```python
from build123d import *

# Parameters (mm, degrees)
F1_DEPTH = 3.048


with BuildPart() as f1:
    # F0 (on Front) → F1 (new body)
    with BuildSketch(Plane.XZ):
        with BuildLine():
            Line((-9.525, 114.3), (-15.7474569047, 65.5082893304))
            ThreePointArc((-15.7474569047, 65.5082893304), (-10.4912828548, 75.4142187767), (0, 79.375))
            Line((0, 79.375), (0, 104.775))
            ThreePointArc((0, 104.775), (-6.7351920908, 107.5648079092), (-9.525, 114.3))
        make_face()
        with BuildLine():
            Line((0, 104.775), (0, 79.375))
            ThreePointArc((0, 79.375), (10.4912828548, 75.4142187767), (15.7474569047, 65.5082893304))
            Line((15.7474569047, 65.5082893304), (9.525, 114.3))
            ThreePointArc((9.525, 114.3), (6.7351920908, 107.5648079092), (0, 104.775))
        make_face()
        with BuildLine():
            ThreePointArc((9.525, 114.3), (0, 123.825), (-9.525, 114.3))
            ThreePointArc((-9.525, 114.3), (-6.7351920908, 107.5648079092), (0, 104.775))
            ThreePointArc((0, 104.775), (6.7351920908, 107.5648079092), (9.525, 114.3))
        make_face()
        with BuildLine():
            ThreePointArc((3.175, 114.3), (2.2450640303, 112.0549359697), (0, 111.125))
            ThreePointArc((0, 111.125), (-2.2450640303, 116.5450640303), (3.175, 114.3))
        make_face(mode=Mode.SUBTRACT)
        with BuildLine():
            ThreePointArc((-15.7474569047, 61.4917106696), (-10.4912828548, 51.5857812233), (0, 47.625))
            Line((0, 47.625), (0, 60.325))
            ThreePointArc((0, 60.325), (-3.175, 63.5), (0, 66.675))
            Line((0, 66.675), (0, 79.375))
            ThreePointArc((0, 79.375), (-10.4912828548, 75.4142187767), (-15.7474569047, 65.5082893304))
            ThreePointArc((-15.7474569047, 65.5082893304), (-15.875, 63.5), (-15.7474569047, 61.4917106696))
        make_face()
        with BuildLine():
            ThreePointArc((-9.525, 0), (-6.7351920908, 6.7351920908), (0, 9.525))
            Line((0, 9.525), (0, 47.625))
            ThreePointArc((0, 47.625), (-10.4912828548, 51.5857812233), (-15.7474569047, 61.4917106696))
            Line((-15.7474569047, 61.4917106696), (-9.525, 0))
        make_face()
        with BuildLine():
            Line((0, 47.625), (0, 9.525))
            ThreePointArc((0, 9.525), (6.7351920908, 6.7351920908), (9.525, 0))
            Line((9.525, 0), (36.5125, 0))
            ThreePointArc((36.5125, 0), (38.8373399243, 5.6126600757), (44.45, 7.9375))
            Line((44.45, 7.9375), (17.9461215627, 7.9375))
            ThreePointArc((17.9461215627, 7.9375), (11.9794807993, 10.6336655463), (10.0597951449, 16.8934512966))
            Line((10.0597951449, 16.8934512966), (15.7474569047, 61.4917106696))
            ThreePointArc((15.7474569047, 61.4917106696), (10.4912828548, 51.5857812233), (0, 47.625))
        make_face()
        with BuildLine():
            ThreePointArc((3.175, 0), (-2.2450640303, -2.2450640303), (0, 3.175))
            Line((0, 3.175), (0, 9.525))
            ThreePointArc((0, 9.525), (-6.7351920908, 6.7351920908), (-9.525, 0))
            ThreePointArc((-9.525, 0), (-6.7351920908, -6.7351920908), (0, -9.525))
            Line((0, -9.525), (0.6794904459, -9.5007324841))
            ThreePointArc((0.6794904459, -9.5007324841), (6.9712901065, -6.4905114784), (9.525, 0))
            Line((9.525, 0), (3.175, 0))
        make_face()
        with BuildLine():
            Line((0, 9.525), (0, 3.175))
            ThreePointArc((0, 3.175), (2.2450640303, 2.2450640303), (3.175, 0))
            Line((3.175, 0), (9.525, 0))
            ThreePointArc((9.525, 0), (6.7351920908, 6.7351920908), (0, 9.525))
        make_face()
        with BuildLine():
            Line((36.5125, 0), (9.525, 0))
            ThreePointArc((9.525, 0), (6.9712901065, -6.4905114784), (0.6794904459, -9.5007324841))
            Line((0.6794904459, -9.5007324841), (44.45, -7.9375))
            ThreePointArc((44.45, -7.9375), (38.8373399243, -5.6126600757), (36.5125, 0))
        make_face()
        with BuildLine():
            ThreePointArc((44.45, 7.9375), (38.8373399243, 5.6126600757), (36.5125, 0))
            ThreePointArc((36.5125, 0), (38.8373399243, -5.6126600757), (44.45, -7.9375))
            ThreePointArc((44.45, -7.9375), (50.0626600757, -5.6126600757), (52.3875, 0))
            ThreePointArc((52.3875, 0), (50.0626600757, 5.6126600757), (44.45, 7.9375))
        make_face()
        with BuildLine():
            ThreePointArc((47.625, 0), (44.45, -3.175), (41.275, 0))
            ThreePointArc((41.275, 0), (44.45, 3.175), (47.625, 0))
        make_face(mode=Mode.SUBTRACT)
        with BuildLine():
            Line((0, 60.325), (0, 47.625))
            ThreePointArc((0, 47.625), (10.4912828548, 51.5857812233), (15.7474569047, 61.4917106696))
            ThreePointArc((15.7474569047, 61.4917106696), (15.8430821396, 62.4938323604), (15.875, 63.5))
            ThreePointArc((15.875, 63.5), (15.8430821396, 64.5061676396), (15.7474569047, 65.5082893304))
            ThreePointArc((15.7474569047, 65.5082893304), (10.4912828548, 75.4142187767), (0, 79.375))
            Line((0, 79.375), (0, 66.675))
            ThreePointArc((0, 66.675), (2.2450640303, 65.7450640303), (3.175, 63.5))
            ThreePointArc((3.175, 63.5), (2.2450640303, 61.2549359697), (0, 60.325))
        make_face()
    extrude(amount=F1_DEPTH)


solid = f1.part
```
Check sheet for the modelled part. Datum: model origin and axes. Units: mm. A direction names the side the tool comes from. Give positions to 0.01 mm unless a question says otherwise; leave off trailing zeros. Write each loop counter-clockwise with the first axis right and the second up, starting at its lowest first coordinate (ties: lowest second). Pieces come first, ordered by that corner, then holes. Notation, with made-up numbers: (-18, 30.25) -> (24, 30.25) arc R11 ccw to (24, 36.25) -> close; hole circle Ø3 at (89, 75). An arc over 180 degrees is marked (long way). Use CSV: the item, a comma, the result in double quotes. Start each with the question number.
Q1. Cross-section at C-C on z = 53. Enter the section's corners in (x, y).
Q2. Release check for a two-part mould opening along Z. For faces 1 (the flat face through (3, -3.048, 43)), 2 (the flat face through (12.864, -1.503, 38.88)), 3 (the flat face through (-12.6, -1.5, 90.2)) record: +Z half, -Z half, draft (parallel to the pull), parting line (faces both ways), or undercut.
Q3. Depth check by flat-ended pin: P1, Ø5, axis at x = 0, z = 114.3, coming from the +Y side. Enter the tip coordinate at first touch or a pass-through.
Q4. Cross-section at B-B on x = 38.5. Enter the section's corners in (y, z), and give its area (3 significant figures).
Q5. Tool access check on faces 4 (the flat face through (31, -2, 7.938)), 5 (the cylindrical face through (41.52, -1.5, -1.22)). Record the directions out of +Z, -Z, +X, -X, +Y, -Y that give a thin tool (end or side, any length) a straight path to the whole face; none if there is none.
Q6. Cross-section at A-A on y = -1.2. Count the separate pieces of the cut face and the enclosed holes in it, and give its area (3 significant figures).
Q7. Scan lines: line 1 along Z through (x, y) = (0, -1.15) (3 decimals); line 2 along X through (y, z) = (-1.5, 114.3) (3 decimals); line 3 along X through (y, z) = (-1.9, 65). Record each from-to range of solid material in increasing order.
Working result:
1,outline,"(-14.89, -3.05) -> (14.66, -3.05) -> (14.66, 0) -> (-14.89, 0) -> close"
2,face 1,"draft"
2,face 2,"undercut"
2,face 3,"+Z half"
3,P1,"passes through"
4,outline,"(-3.05, -8.15) -> (0, -8.15) -> (0, 7.94) -> (-3.05, 7.94) -> close"
4,area,"49.0 mm^2"
5,face 4,"+Z, +X, +Y, -Y"
5,face 5,"+Y, -Y"
6,separate pieces,"1"
6,enclosed holes,"4"
6,area,"3,740 mm^2"
7,line 1,"z = -9.525 to -3.175, 3.175 to 60.325, 66.675 to 111.125, 117.475 to 123.825"
7,line 2,"x = -9.525 to -3.175, 3.175 to 9.525"
7,line 3,"x = -15.8 to -2.8, 2.8 to 15.8"
